```python
from build123d import *

# Parameters (mm, degrees)
BOSS_EXTRUDE1_DEPTH = 4.3
CUT_EXTRUDE1_START  = -5.3
SKETCH2_W           = 3
SKETCH2_H           = 17
SKETCH2_W_2         = 4.3
SKETCH2_H_2         = 16.2
CUT_EXTRUDE1_DEPTH  = 6.3


with BuildPart() as part:
    # Sketch1 → Boss-Extrude1 (new body)
    with BuildSketch(Plane(origin=(0, 0, 0), x_dir=(1, 0, 0), z_dir=(0, 1, 0))):
        Polygon((335.3, -13.5), (762, 17.8), (762, 37.8), (335.3, 13.5), (0, 13.5), (0, -13.5), align=None)
    boss_extrude1 = extrude(amount=BOSS_EXTRUDE1_DEPTH)

    # Sketch2 → Cut-Extrude1 (cut)
    with BuildSketch(Plane(origin=(0, 4.3, 0), x_dir=(1, 0, 0), z_dir=(0, 1, 0)).offset(CUT_EXTRUDE1_START)):
        with Locations((81.5, -5)):
            Rectangle(SKETCH2_W, SKETCH2_H)
        with Locations((150.5, -5)):
            Rectangle(SKETCH2_W, SKETCH2_H)
        with Locations((219.5, -5)):
            Rectangle(SKETCH2_W, SKETCH2_H)
        with Locations((288.5, -5)):
            Rectangle(SKETCH2_W, SKETCH2_H)
        with Locations((550.81, 10.250733536)):
            Rectangle(SKETCH2_W_2, SKETCH2_H_2)
    cut_extrude1 = extrude(amount=CUT_EXTRUDE1_DEPTH, mode=Mode.SUBTRACT)

    # Mirror1: Boss-Extrude1, Cut-Extrude1 across plane
    add(boss_extrude1.mirror(Plane(origin=(0, 0, 0), x_dir=(0, 0, 1), z_dir=(1, 0, 0))))
    add(cut_extrude1.mirror(Plane(origin=(0, 0, 0), x_dir=(0, 0, 1), z_dir=(1, 0, 0))), mode=Mode.SUBTRACT)


solid = part.part
```
For this review, take the finished solid that the model builds, in its own axes (mm). A direction names the side the tool comes from. Round coordinates to 2 decimals unless told otherwise and drop trailing zeros. Write each loop counter-clockwise with the first axis right and the second up, starting at its lowest first coordinate (ties: lowest second). Pieces come first, ordered by that corner, then holes. Notation, with made-up numbers: (19, 23) - (53, 23) arc R27 cw to (53, 58) - close; hole circle Ø10 at (-27, -6). An arc over 180 degrees is marked (long way). Use CSV: the item, a comma, the result in double quotes.
1) Add section B-B on x = -648. Write out the cut boundary in (y, z).
Conclusion:
outline,"(0, -31.31) - (4.3, -31.31) - (4.3, -9.44) - (0, -9.44) - close"
2) For faces 1 (the flat face through (11, 4.3, -7)), 2 (the flat face through (-551.64, 2.12, -25.82)), list the 3-axis set-ups (+Z, -Z, +X, -X, +Y, -Y) from which the entire face can be reached by the end or side of a thin tool; tool diameter is ignored.
Conclusion:
face 1,"+Z, -Z, +X, -X, +Y"
face 2,"-Z, +Y, -Y"
3) Add section A-A on x = 321. Write out the cut boundary in (y, z).
Conclusion:
outline,"(0, -13.5) - (4.3, -13.5) - (4.3, 13.5) - (0, 13.5) - close"
4) Wall thickness on line 1 along Z through (x, y) = (88.5, 0.4); line 2 along Z through (x, y) = (615, 1.9): over which ranges is each line inside the solid? List them lowest first. Write a range as from..to.
Conclusion:
line 1,"z = -13.5..13.5"
line 2,"z = -29.43..-7.02"
5) Clearance check with flat-ended pins moving along their axes: pin 1 Ø1.5 at (x, y) = (-220, 1) entering from +Z; pin 2 Ø2 at (x, y) = (-434.5, 1.5) entering from -Z; pin 3 Ø5 at (x, z) = (-473, -26) entering from +Y; pin 4 Ø1.3 at (x, y) = (-550.5, 3) entering from +Z. State where each tip first meets the part, or that it passes through.
Conclusion:
pin 1,"stops at z = -3.5"
pin 2,"stops at z = -19.21"
pin 3,"passes through"
pin 4,"stops at z = -18.35"
